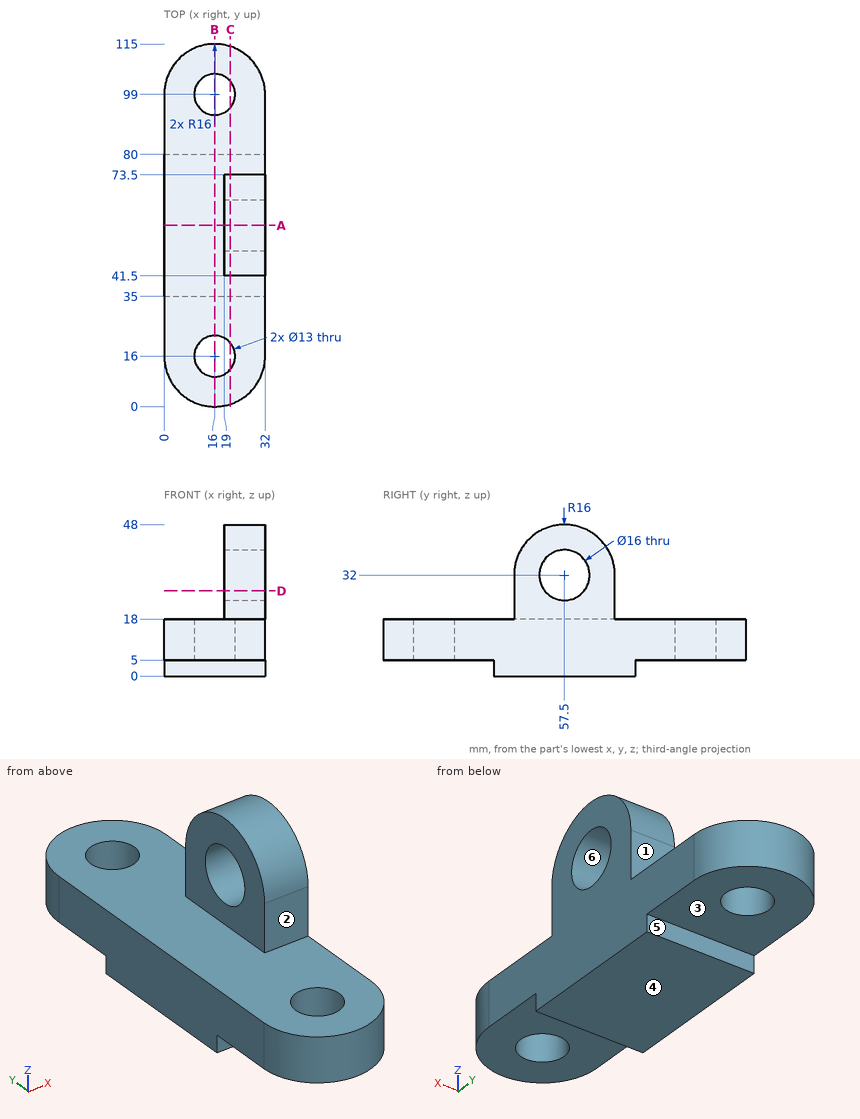
Answer from the drawing. Dimensions are ordinates in mm from the lowest x, y and z of the part. A direction names the side the tool comes from. Give positions to 0.01 mm unless a question says otherwise; leave off trailing zeros. Write each loop counter-clockwise with the first axis right and the second up, starting at its lowest first coordinate (ties: lowest second). Pieces come first, ordered by that corner, then holes.
1) Section B-B (x = 16) is taken. Write down the section's boundary in (y, z), and give its area (3 significant figures).
2) For a pull along Z with two mould halves and no side action, classify the marked faces 4, 5 and 6 as pulls with the +Z half, pulls with the -Z half, needs draft (parallel to the pull), parting line crosses it, or undercut.
3) Section D-D (z = 27) is taken. Write down the section's boundary in (x, y) (3 decimals).
4) Section C-C (x = 21) is taken. Write down the section's boundary in (y, z), and give its area (3 significant figures).
5) Find the intervals of material crossed by L1, parallel to Y at x = 16, z = 13.5; L2, parallel to Z at x = 25, y = 57; L3, parallel to Z at x = 15, y = 42.5, in increasing order.
6) A tool of negligible diameter and unlimited length cuts with its end or side. For the marked faces 1, 2 and 3, from which of +Z, -Z, +X, -X, +Y, -Y can it reach the whole face along a straight path? Write none if from no direction.
7) Given P1, Ø1.5, axis at x = 18, z = 2.5, coming from the +Y side; P2, Ø12, axis at x = 25, z = 17, coming from the -Y side; P3, Ø1.5, axis at x = 8.5, z = 13.5, coming from the +Y side; P4, Ø8, axis at x = 16, y = 99, coming from the -Z side, each flat-ended and moving along its own axis, determine where each tip first touches the part or whether it passes through.
8) Section A-A (y = 57.5) is taken. Write down the section's boundary in (x, z), and give its area (3 significant figures).
Response:
1. outline: (0, 5) - (9.5, 5) - (9.5, 18) - (0, 18) - close; (22.5, 5) - (35, 5) - (35, 0) - (80, 0) - (80, 5) - (92.5, 5) - (92.5, 18) - (22.5, 18) - close; (105.5, 5) - (115, 5) - (115, 18) - (105.5, 18) - close
1. area: 1,380 mm2
2. face 4: pulls with the -Z half
2. face 5: needs draft
2. face 6: undercut
3. outline: (19, 41.5) - (32, 41.5) - (32, 51.255) - (19, 51.255) - close; (19, 63.745) - (32, 63.745) - (32, 73.5) - (19, 73.5) - close
4. outline: (0.8, 5) - (11.85, 5) - (11.85, 18) - (0.8, 18) - close; (20.15, 5) - (35, 5) - (35, 0) - (80, 0) - (80, 5) - (94.85, 5) - (94.85, 18) - (73.5, 18) - (73.5, 32) arc R16 ccw to (41.5, 32) - (41.5, 18) - (20.15, 18) - close; (103.15, 5) - (114.2, 5) - (114.2, 18) - (103.15, 18) - close; hole circle Ø16 at (57.5, 32)
4. area: 2,130 mm2
5. L1: y = 0 to 9.5, 22.5 to 92.5, 105.5 to 115
5. L2: z = 0 to 24.02, 39.98 to 47.99
5. L3: z = 0 to 18
6. face 1: +Z, +X, -X, +Y
6. face 2: +Z, +X, -X, -Y
6. face 3: -Z, +X, -X, +Y
7. P1: stops at y = 80
7. P2: stops at y = 0.28
7. P3: stops at y = 113.51
7. P4: passes through
8. outline: (0, 0) - (32, 0) - (32, 24) - (19, 24) - (19, 18) - (0, 18) - close; (19, 40) - (32, 40) - (32, 48) - (19, 48) - close
8. area: 758 mm2
